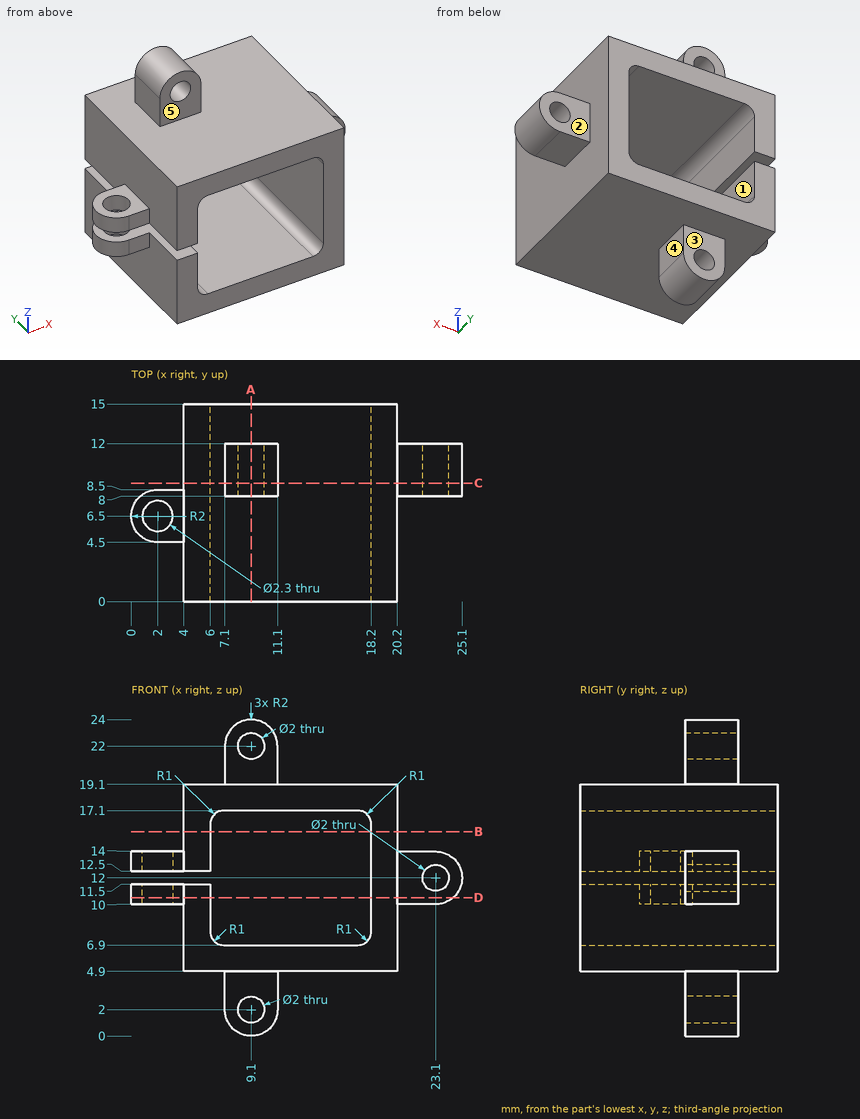
Print and shaded views of the part. All mm, measured from the part's lowest x, y and z. A direction names the side the tool comes from. Round coordinates to 2 decimals unless told otherwise and drop trailing zeros. Order: outer loops, then holes, each group sorted by start corner. A loop starts at its lowest first (then second) coordinate and runs counter-clockwise, first axis right, second up.
Q1. Slice it at C-C (y = 9). State how many separate pieces and enclosed holes the cut face has, and give its area (3 significant figures).
Q2. Slice it at D-D (z = 10.5). Write the cut outline in (x, y), and give its area (3 significant figures).
Q3. Which spindle directions (+Z, -Z, +X, -X, +Y, -Y) get a long thin tool onto all of the face, cutting with end or side? Do the marked faces 1, 2, 3, 4 and 5. Say none if no direction does.
Q4. Drop flat-ended pins along their axis: pin 1 (3 mm diameter, centred on y = 10, z = 3.5, fed in from -X); pin 2 (4.5 mm diameter, centred on x = 12.5, y = 9.5, fed in from -Z); pin 3 (0.9 mm diameter, centred on y = 10.5, z = 3, fed in from +X); pin 4 (3 mm diameter, centred on x = 10, y = 9.5, fed in from -Z). Give the stop position or say it passes through.
Q5. Slice it at B-B (z = 15.5). Write the cut outline in (x, y).
Q6. Slice it at A-A (x = 9.1). Write the cut outline in (y, z), and give its area (3 significant figures).
Q7. Wall check: L1, parallel to Y at x = 2, z = 13.5; L2, parallel to Z at x = 14.5, y = 6.75; L3, parallel to X at y = 4, z = 14.75. Give the ranges that are in metal, low to high.
Results below:
1. separate pieces: 1
1. enclosed holes: 3
1. area: 149 mm2
2. outline: (2, 4.5) - (4, 4.5) - (4, 0) - (6, 0) - (6, 15) - (4, 15) - (4, 8.5) - (2, 8.5) arc R2 ccw to start; (18.2, 0) - (20.2, 0) - (20.2, 8) - (24.42, 8) - (24.42, 12) - (20.2, 12) - (20.2, 15) - (18.2, 15) - close; hole circle Ø2.3 at (2, 6.5)
2. area: 87.0 mm2
3. face 1: +Y, -Y
3. face 2: +Z, -Z, +X, +Y
3. face 3: -Z, +X, -X, +Y
3. face 4: -Z, +X, +Y, -Y
3. face 5: +Z, +X, -X, -Y
4. pin 1: stops at x = 4
4. pin 2: stops at z = 0.36
4. pin 3: stops at x = 11.1
4. pin 4: stops at z = 0
5. outline: (4, 0) - (6, 0) - (6, 15) - (4, 15) - close; (18.2, 0) - (20.2, 0) - (20.2, 15) - (18.2, 15) - close
6. outline: (0, 4.9) - (8, 4.9) - (8, 3) - (12, 3) - (12, 4.9) - (15, 4.9) - (15, 6.9) - (0, 6.9) - close; (0, 17.1) - (15, 17.1) - (15, 19.1) - (12, 19.1) - (12, 21) - (8, 21) - (8, 19.1) - (0, 19.1) - close; (8, 0) - (12, 0) - (12, 1) - (8, 1) - close; (8, 23) - (12, 23) - (12, 24) - (8, 24) - close
6. area: 83.2 mm2
7. L1: y = 4.5 to 5.35, 7.65 to 8.5
7. L2: z = 4.9 to 6.9, 17.1 to 19.1
7. L3: x = 4 to 6, 18.2 to 20.2
